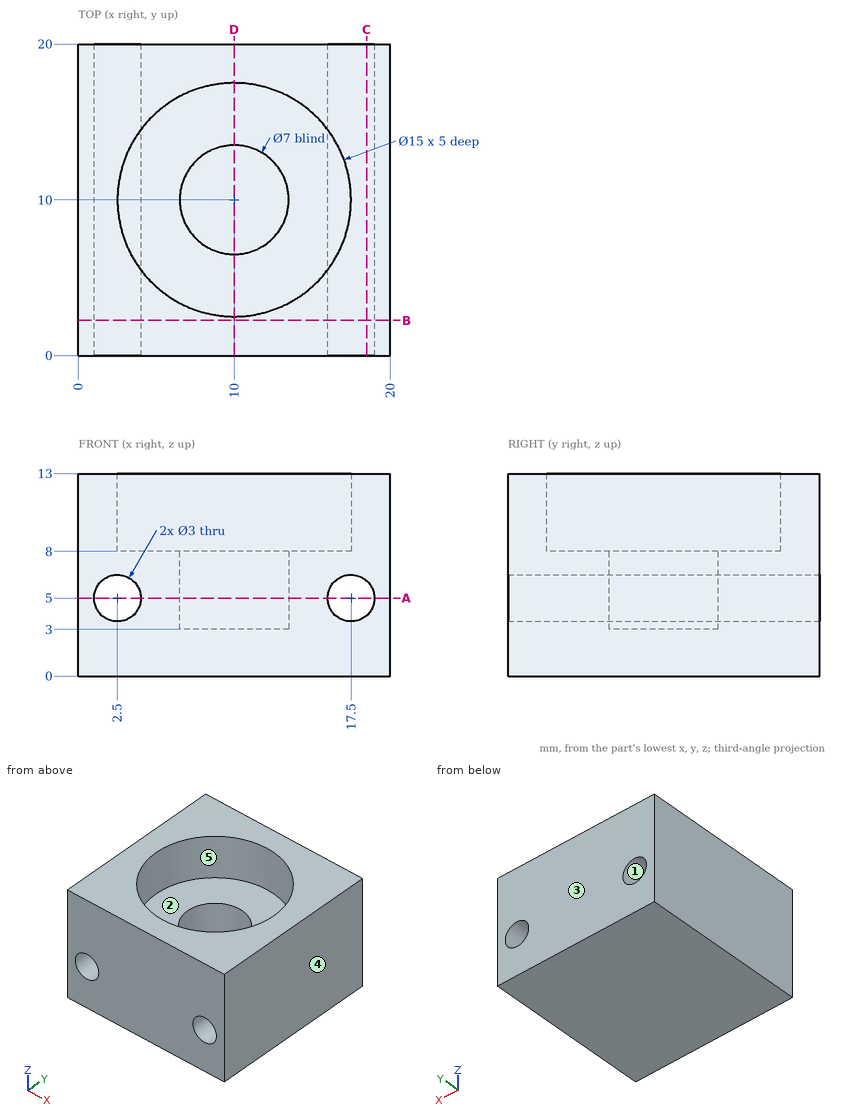
The figure shows three views and two pictorial views of one solid part (mm, origin at its lowest corner). Answer the questions. A direction names the side the tool comes from. Round coordinates to 2 decimals unless told otherwise and drop trailing zeros. Write each loop counter-clockwise with the first axis right and the second up, starting at its lowest first coordinate (ties: lowest second). Pieces come first, ordered by that corner, then holes. Notation, with made-up numbers: M -5,-1.75 L 35,-1.75 A21 ccw 35,36.25 Z; hole C 43.25,-9 d6. An arc over 180 degrees is marked long. Write each question's results on one line, items separated by ' | '. Start each with the question number.
(1) Determine the mould class of the marked faces 1, 2 and 3 for opening direction Z: +Z half, -Z half, draft (parallel to the pull), parting line (faces both ways), or undercut.
(2) The part is cut by section C-C, the plane x = 18.5. Write down the section's boundary in (y, z), and give its area (3 significant figures).
(3) For the marked faces 4 and 5, determine the directions among +Z, -Z, +X, -X, +Y, -Y from which every point of the face is accessible in a straight line to the end or side of a thin tool.
(4) Find the intervals of material crossed by line 1 (Y direction, x = 14.5, z = 9); line 2 (X direction, y = 9.75, z = 9.5); line 3 (X direction, y = 16.5, z = 10.75), in increasing order.
(5) Each of these flat-tipped pins is pushed along its axis until it touches: P1, Ø3.5, axis at x = 11, y = 11, coming from the +Z side; P2, Ø4.5, axis at x = 9, y = 6.5, coming from the +Z side; P3, Ø1.8, axis at x = 17.5, z = 5, coming from the +Y side. Where does it stop, or does it pass through?
(6) The part is cut by section B-B, the plane y = 2.25. Write down the section's boundary in (x, z), and give its area (3 significant figures).
(7) The part is cut by section A-A, the plane z = 5. Write down the section's boundary in (x, y), and give its area (3 significant figures).
(8) The part is cut by section D-D, the plane x = 10. Write down the section's boundary in (y, z), and give its area (3 significant figures).
Worked answers:
1) face 1: undercut | face 2: +Z half | face 3: draft
2) outline: M 0,0 L 20,0 L 20,3.88 L 0,3.88 Z; M 0,6.12 L 20,6.12 L 20,13 L 0,13 Z | area: 215 mm²
3) face 4: +Z, -Z, +X, +Y, -Y | face 5: +Z
4) line 1: y = 0 to 4, 16 to 20 | line 2: x = 0 to 2.5, 17.5 to 20 | line 3: x = 0 to 6.26, 13.74 to 20
5) P1: stops at z = 3 | P2: stops at z = 8 | P3: passes through
6) outline: M 0,0 L 20,0 L 20,13 L 0,13 Z; hole C 2.5,5 d3; hole C 17.5,5 d3 | area: 246 mm²
7) outline: M 0,0 L 1,0 L 1,20 L 0,20 Z; M 4,0 L 16,0 L 16,20 L 4,20 Z; M 19,0 L 20,0 L 20,20 L 19,20 Z; hole C 10,10 d7 | area: 242 mm²
8) outline: M 0,0 L 20,0 L 20,13 L 17.5,13 L 17.5,8 L 13.5,8 L 13.5,3 L 6.5,3 L 6.5,8 L 2.5,8 L 2.5,13 L 0,13 Z | area: 150 mm²
